Design review of the part built by this model. Coordinates are the model's own, in mm. Face numbers are marked on the shaded views. A direction names the side the tool comes from. Coordinates: 2 decimals unless noted, no trailing zeros. Write each loop counter-clockwise with the first axis right and the second up, starting at its lowest first coordinate (ties: lowest second). Pieces come first, ordered by that corner, then holes. Notation, with made-up numbers: (31, 36) -> (57, 36) arc R26 ccw to (57, 51) -> close; hole circle Ø11 at (54, -30.75). An arc over 180 degrees is marked (long way). Answer in a Markdown table with one row per item. Add a question column.
Item 1: Take a section at A-A, the plane z = -76. Write out the cut boundary in (x, y).
Item 2: Clearance check with flat-ended pins moving along their axes: P1, Ø3, axis at y = 9.5, z = -54, coming from the +X side; P2, Ø7.5, axis at x = -52, z = -170.5, coming from the -Y side; P3, Ø5, axis at y = 30.5, z = -147, coming from the -X side. State where each tip first meets the part, or that it passes through.
Item 3: To check wall thickness, follow line 1 (Z direction, x = -5, y = 43); line 2 (X direction, y = 82, z = -93); line 3 (Z direction, x = -36.5, y = 69.5). State the ranges of each line that lie inside material, in increasing order.
Item 4: Take a section at D-D, the plane y = 74. Write out the cut boundary in (x, z), and give its area (3 significant figures).
Item 5: Draft analysis for pull direction Z (two halves, no side actions). For the marked faces 4, 5 and 6, state which applies: released by +Z, released by -Z, zero draft, split by the parting line, or undercut.
Item 6: Take a section at B-B, the plane x = -50. Write out the cut boundary in (y, z).
Item 7: For the marked faces 1, 2 and 3, list the 3-axis set-ups (+Z, -Z, +X, -X, +Y, -Y) from which the entire face can be reached by the end or side of a thin tool; tool diameter is ignored.
Item 8: Take a section at C-C, the plane y = 18. Write out the cut boundary in (x, z), and give its area (3 significant figures).
Autodesk Inventor part; units mm, degrees
ref_plane "YZ Plane" through (0, 0, 0) normal (1, 0, 0) x (0, 1, 0)
ref_plane "XZ Plane" through (0, 0, 0) normal (0, 1, 0) x (-1, 0, 0)
ref_plane "XY Plane" through (0, 0, 0) normal (0, 0, 1) x (1, 0, 0)
sketch "Sketch1" plane through (0, 0, 0) normal (0, 1, 0) x (-1, 0, 0)
  line L0 (0, 0) -> (15, 0)
  line L1 (15, 0) -> (15, -15)
  line L2 (15, -15) -> (0, -15)
  line L3 (0, -15) -> (0, 0)
  line L4 (15, -165) -> (0, -165)
  line L5 (0, -165) -> (0, -180)
  line L6 (0, -180) -> (15, -180)
  line L7 (15, -180) -> (15, -165)
  line L8 (65, -180) -> (80, -180)
  line L9 (80, -180) -> (80, -165)
  line L10 (80, -165) -> (65, -165)
  line L11 (65, -165) -> (65, -180)
  line L12 (80, -15) -> (65, -15)
  line L13 (65, -15) -> (65, 0)
  line L14 (65, 0) -> (80, 0)
  line L15 (80, 0) -> (80, -15)
  point P0 (15, -7.5)
  dimension "d0" = 15
  dimension "d1" = 15
  dimension "d2" = 15
  dimension "d3" = 15
  dimension "d4" = 15
  dimension "d5" = 15
  dimension "d6" = 150
  dimension "d7" = 50
extrude "Extrusion1" add sketch "Sketch1" along normal blind 5
sketch "Sketch2" plane through (0, 5, 0) normal (0, 1, 0) x (1, 0, 0)
  line L0 (-80, 0) -> (-65, 0)
  line L1 (-80, 0) -> (-65, 0)
  line L2 (-65, 0) -> (-65, 180)
  line L3 (-65, 180) -> (-80, 180)
  line L4 (-80, 180) -> (-80, 0)
  line L5 (-15, 165) -> (0, 165)
  line L6 (-65, 180) -> (0, 180)
  line L7 (0, 180) -> (0, 165)
  line L8 (0, 165) -> (-65, 165)
  line L9 (-65, 165) -> (-65, 180)
  line L10 (-15, 0) -> (0, 0)
  line L11 (-15, 165) -> (0, 165)
  line L12 (0, 165) -> (0, 0)
  line L13 (0, 0) -> (-15, 0)
  line L14 (-15, 0) -> (-15, 165)
  line L15 (-15, 0) -> (-65, 0)
  line L16 (-65, 0) -> (-65, 15)
  line L17 (-65, 15) -> (-15, 15)
  line L18 (-15, 15) -> (-15, 0)
  point P0 (-65, 165)
extrude "Extrusion2" add sketch "Sketch2" along normal blind 80 contours L4 L3 L2 L0 | L2 L17 L14 L15 | L14 L5 L12 L10 | L6 L7 L5 L8 L2
sketch "Sketch3" plane through (0, 85, 0) normal (0, 1, 0) x (1, 0, 0)
  line L0 (-90, -10) -> (10, -10)
  line L1 (10, -10) -> (10, 190)
  line L2 (10, 190) -> (-90, 190)
  line L3 (-90, 190) -> (-90, -10)
  line L4 (-80, 180) -> (-80, 0)
  line L5 (0, 180) -> (-80, 180)
  line L6 (0, 0) -> (0, 180)
  line L7 (-80, 0) -> (0, 0)
  point P0 (-40, -10)
  dimension "d12" = 10
  dimension "d13" = 10
  dimension "d14" = 10
  dimension "d15" = 10
extrude "Extrusion3" add sketch "Sketch3" along normal blind 5 contours L3 L2 L1 L0 | L5 L6 L7 L4
fillet "Fillet1" radius 30 4 edges at (10, 87.5, 10) (-90, 87.5, 10) (-90, 87.5, -190) (10, 87.5, -190)
sketch "Sketch4" plane through (0, 0, 0) normal (1, 0, 0) x (0, 0, -1)
  line L0 (160, 5) -> (130, 5)
  line L1 (130, 5) -> (130, 65)
  line L2 (130, 65) -> (160, 65)
  line L3 (160, 65) -> (160, 5)
  line L4 (25, 70) -> (85, 70)
  line L5 (85, 70) -> (85, 30)
  line L6 (85, 30) -> (25, 30)
  line L7 (25, 30) -> (25, 70)
  line L8 (0, 0) -> (0, 85)
  line L9 (180, 0) -> (180, 85)
  line L10 (15, 5) -> (165, 5)
  line L11 (20, 85) -> (160, 85)
  line L12 (52.5, 70) -> (57.5, 70)
  line L13 (57.5, 70) -> (57.5, 30)
  line L14 (57.5, 30) -> (52.5, 30)
  line L15 (52.5, 30) -> (52.5, 70)
  line L16 (85, 52.5) -> (25, 52.5)
  line L17 (25, 52.5) -> (25, 47.5)
  line L18 (25, 47.5) -> (85, 47.5)
  line L19 (85, 47.5) -> (85, 52.5)
  point P0 (52.5, 52.5)
  point P1 (52.5, 47.5)
  point P2 (57.5, 47.5)
  point P3 (57.5, 52.5)
  dimension "d19" = 60
  dimension "d20" = 30
  dimension "d21" = 40
  dimension "d22" = 60
  dimension "d23" = 25
  dimension "d24" = 20
  dimension "d25" = 0
  dimension "d26" = 15
  dimension "d27" = 5
  dimension "d28" = 5
  dimension "d29" = 17.5
  dimension "d30" = 27.5
extrude "Extrusion4" cut sketch "Sketch4" against normal blind 15 contours L0 L1 L2 L3 | L4 L15 L16 L7 | L4 L5 L16 L13 | L18 L15 L6 L7 | L18 L5 L6 L13
properties part number "huis"
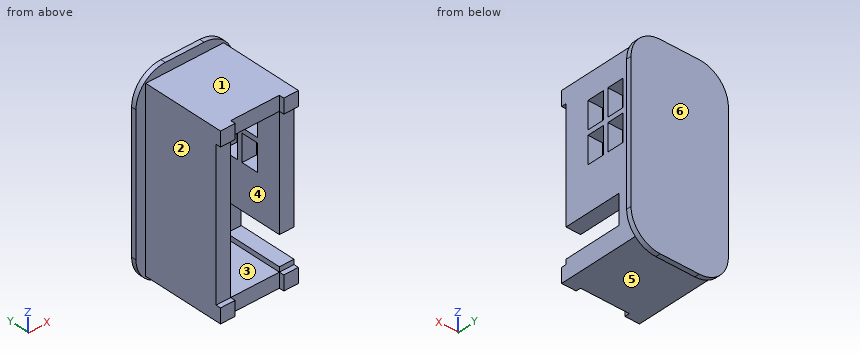
Answers:
| question | item | result |
|---|---|---|
| 1 | outline | (-90, 85) -> (-80, 85) -> (-80, 5) -> (-65, 5) -> (-65, 85) -> (-15, 85) -> (-15, 70) -> (0, 70) -> (0, 85) -> (10, 85) -> (10, 90) -> (-90, 90) -> close; (-15, 5) -> (0, 5) -> (0, 30) -> (-15, 30) -> close; (-15, 47.5) -> (0, 47.5) -> (0, 52.5) -> (-15, 52.5) -> close |
| 2 | P1 | stops at x = 0 |
| 2 | P2 | stops at y = 5 |
| 2 | P3 | stops at x = -80 |
| 3 | line 1 | z = -180 to -160, -130 to -85, -57.5 to -52.5, -25 to 0 |
| 3 | line 2 | x = -80 to -65, -15 to 0 |
| 3 | line 3 | z = -180 to -165, -15 to 0 |
| 4 | outline | (-80, -180) -> (0, -180) -> (0, 0) -> (-80, 0) -> close; hole (-65, -165) -> (-15, -165) -> (-15, -15) -> (-65, -15) -> close |
| 4 | area | 6,900 mm^2 |
| 5 | face 4 | undercut |
| 5 | face 5 | released by -Z |
| 5 | face 6 | zero draft |
| 6 | outline | (5, -180) -> (85, -180) -> (85, -190) -> (90, -190) -> (90, 10) -> (85, 10) -> (85, 0) -> (5, 0) -> (5, -15) -> (85, -15) -> (85, -165) -> (5, -165) -> close |
| 7 | face 1 | +Z, +X, -X, -Y |
| 7 | face 2 | +Z, -Z, -X, -Y |
| 7 | face 3 | -Y |
| 8 | outline | (-80, -180) -> (0, -180) -> (0, -160) -> (-15, -160) -> (-15, -165) -> (-65, -165) -> (-65, -15) -> (-15, -15) -> (-15, -130) -> (0, -130) -> (0, 0) -> (-80, 0) -> close |
| 8 | area | 6,450 mm^2 |
